Geometry check sheet. Reference: the model listing, model coordinates, mm. Face numbers are marked on the shaded views. A direction names the side the tool comes from. Give positions to 0.01 mm unless a question says otherwise; leave off trailing zeros. Loops run counter-clockwise (first coordinate to the right, second up) from the corner with the lowest first, then second, coordinate; pieces in that order, holes last. Notation, with made-up numbers: (19.25, 70) -> (38.25, 70) arc R33 ccw to (38.25, 103) -> close; hole circle Ø5 at (-20, 60.5). An arc over 180 degrees is marked (long way). One line per item, written item: value. Start each with the question number.
(1) Sectioned sample at D-D, the plane z = 0. Record the cut outline in (x, y).
(2) Draft check along Z on the marked faces 1, 2 and 3. Enter one of: pulls with the +Z half, pulls with the -Z half, needs draft (parallel to the pull), parting line crosses it, or undercut.
(3) Gauge pin test, flat ends, axial feed: pin 1 Ø4 at (x, z) = (-20, -10.5) entering from +Y; pin 2 Ø16.5 at (y, z) = (18, 32.5) entering from -X; pin 3 Ø20.5 at (x, z) = (-11, 43.5) entering from +Y (3 decimals). Record the tip position at first contact, or that the pin passes through.
(4) Sectioned sample at B-B, the plane y = 25.5. Record the cut outline in (x, z) (3 decimals).
(5) Tool access check on the marked faces 4 and 5. Record the directions out of +Z, -Z, +X, -X, +Y, -Y that give a thin tool (end or side, any length) a straight path to the whole face; none if there is none.
(6) Sectioned sample at C-C, the plane x = 0. Record the cut outline in (y, z) (3 decimals).
(7) Sectioned sample at A-A, the plane z = 33.02. Record the cut outline in (x, y) (1 decimal).
(8) Scan lines: line 1 along X through (y, z) = (13.5, 32) (3 decimals); line 2 along Z through (x, y) = (70.5, 17.5); line 3 along Y through (x, z) = (-58.5, -22.5). Record each from-to range of solid material in increasing order. Write a range as from..to.
from build123d import *

# Parameters (mm, degrees)
EXTRUDE_THIN1_DEPTH             = 50.8
FILLET1_RADIUS                  = 4.7625
FILLET1_LENGTH                  = 50.8
FILLET2_R                       = 2.54
CUT_EXTRUDE1_DEPTH              = 97.928543268
CUT_EXTRUDE1_DEPTH_BACK         = 97.928543268
SKETCH5_W                       = 25.4
SKETCH5_H                       = 22.733
CUT_EXTRUDE3_START              = -76.2
SKETCH8_W                       = 50.8
SKETCH8_H                       = 31.75
CUT_EXTRUDE3_DEPTH              = 0.508
M6X1_0_TAPPED_HOLE1_D           = 5
M6X1_0_TAPPED_HOLE1_CSINK_D     = 6.05
M6X1_0_TAPPED_HOLE1_CSINK_ANGLE = 90
MIRROR1_START                   = -50.8
MIRROR1_OUTLINE_W               = 151.384
MIRROR1_OUTLINE_H               = 9.017
MIRROR1_DEPTH                   = 101.6
MIRROR1_2_DEPTH                 = 15.2799999
MIRROR1_START_2                 = 35.5200001
MIRROR1_3_DEPTH                 = 15.2799999
MIRROR1_START_3                 = -30.5199999
MIRROR1_4_DEPTH                 = 5.1199999
MIRROR1_START_4                 = 25.4
MIRROR1_5_DEPTH                 = 5.1199999
MIRROR1_START_5                 = -35.5200001
MIRROR1_6_DEPTH                 = 5.0000002
MIRROR1_START_6                 = 30.5199999
MIRROR1_7_DEPTH                 = 5.0000002
CUT_EXTRUDE2_DEPTH              = 97.529691619
CUT_EXTRUDE2_DEPTH_BACK         = 97.529691619
SKETCH7_R                       = 19.05
M4X0_7_TAPPED_HOLE3_D           = 3.3
M4X0_7_TAPPED_HOLE3_CSINK_D     = 5
M4X0_7_TAPPED_HOLE3_CSINK_ANGLE = 90


with BuildPart() as part:
    # Sketch4 → Extrude-Thin1 (new body)
    with BuildSketch(Plane.XY):
        Polygon((0, 0), (-76.2, 0), (-76.2, 31.75), (-66.675, 31.75), (-66.675, 9.525), (0, 9.525), align=None)
    extrude(amount=EXTRUDE_THIN1_DEPTH)

    # Fillet1: full round fillet: the end face becomes a half cylinder, R = half its width
    fillet1_face = Plane((-71.4375, 31.75, 25.4), x_dir=(0, 0, -1), z_dir=(0, 1, 0))  # on the end face: x along it, z out of the body
    fillet1_slab = fillet1_face.offset(-FILLET1_RADIUS / 2) * Box(FILLET1_LENGTH, 2 * FILLET1_RADIUS, FILLET1_RADIUS, mode=Mode.PRIVATE)  # the body's end, R deep
    fillet1_round = Plane((-71.4375, 26.9875, 25.4), x_dir=(0, 1, 0), z_dir=(0, 0, -1)) * Cylinder(FILLET1_RADIUS, FILLET1_LENGTH, mode=Mode.PRIVATE)  # its axis R under the face
    add(fillet1_slab - fillet1_round, mode=Mode.SUBTRACT)

    # Fillet2
    fillet2_edges = [part.edges().sort_by_distance(p)[0] for p in [
        (-66.675, 9.525, 25.4),
    ]]
    fillet(fillet2_edges, radius=FILLET2_R)

    # Sketch5 → Cut-Extrude1 (cut, two sides: drawn at the far end of the back side and taken through both)
    with BuildSketch(Plane(origin=(0, 0, 0), x_dir=(0, 0, -1), z_dir=(1, 0, 0)).offset(-CUT_EXTRUDE1_DEPTH_BACK)):
        with Locations((-12.7, 20.3835)):
            Rectangle(SKETCH5_W, SKETCH5_H)
    extrude(amount=CUT_EXTRUDE1_DEPTH + CUT_EXTRUDE1_DEPTH_BACK, mode=Mode.SUBTRACT)

    # Sketch8 → Cut-Extrude3 (cut)
    with BuildSketch(Plane(origin=(0, 0, 0), x_dir=(0, 0, -1), z_dir=(1, 0, 0)).offset(CUT_EXTRUDE3_START)):
        with Locations((-25.4, 15.875)):
            Rectangle(SKETCH8_W, SKETCH8_H)
    extrude(amount=CUT_EXTRUDE3_DEPTH, mode=Mode.SUBTRACT)

    # M6x1.0 Tapped Hole1 (through all)
    with Locations(Plane.ZY.offset(75.692)):
        with Locations((33.02, 17.145)):
            CounterSinkHole(M6X1_0_TAPPED_HOLE1_D / 2, M6X1_0_TAPPED_HOLE1_CSINK_D / 2, counter_sink_angle=M6X1_0_TAPPED_HOLE1_CSINK_ANGLE)

    # Mirror1: read off the stored shape, not the designer's step
    # Mirror1 outline → Mirror1 (add)
    with BuildSketch(Plane.XY.offset(MIRROR1_START)):
        with Locations((0, 4.5085)):
            Rectangle(MIRROR1_OUTLINE_W, MIRROR1_OUTLINE_H)
    extrude(amount=MIRROR1_DEPTH)

    # Mirror1 2 outline → Mirror1 2 (add)
    with BuildSketch(Plane.XY.offset(MIRROR1_START)):
        with BuildLine():
            Line((-66.675, 12.065), (-66.675, 26.9875))
            ThreePointArc((-66.675, 26.9875), (-70.337647737, 31.621259947), (-75.692, 29.127742042))
            Line((-75.692, 29.127742042), (-75.692, 9.017))
            Line((-75.692, 9.017), (75.692, 9.017))
            Line((75.692, 9.017), (75.692, 29.127742042))
            ThreePointArc((75.692, 29.127742042), (70.337647737, 31.621259947), (66.675, 26.9875))
            Line((66.675, 26.9875), (66.675, 12.065))
            ThreePointArc((66.675, 12.065), (65.931051224, 10.268948776), (64.135, 9.525))
            Line((64.135, 9.525), (-64.135, 9.525))
            ThreePointArc((-64.135, 9.525), (-65.931051224, 10.268948776), (-66.675, 12.065))
        make_face()
    extrude(amount=MIRROR1_2_DEPTH)

    # Mirror1 3 outline → Mirror1 3 (add)
    with BuildSketch(Plane.XY.offset(MIRROR1_START_2)):
        with BuildLine():
            Line((0, 9.525), (0, 9.017))
            Line((0, 9.017), (75.692, 9.017))
            Line((75.692, 9.017), (75.692, 29.127742042))
            ThreePointArc((75.692, 29.127742042), (70.337647737, 31.621259947), (66.675, 26.9875))
            Line((66.675, 26.9875), (66.675, 12.065))
            ThreePointArc((66.675, 12.065), (65.931051224, 10.268948776), (64.135, 9.525))
            Line((64.135, 9.525), (0, 9.525))
        make_face()
    extrude(amount=MIRROR1_3_DEPTH)

    # Mirror1 4 outline → Mirror1 4 (add)
    with BuildSketch(Plane.XY.offset(MIRROR1_START_3)):
        with BuildLine():
            Line((-66.675, 12.065), (-66.675, 26.9875))
            ThreePointArc((-66.675, 26.9875), (-70.337647737, 31.621259947), (-75.692, 29.127742042))
            Line((-75.692, 29.127742042), (-75.692, 9.017))
            Line((-75.692, 9.017), (75.692, 9.017))
            Line((75.692, 9.017), (75.692, 29.127742042))
            ThreePointArc((75.692, 29.127742042), (70.337647737, 31.621259947), (66.675, 26.9875))
            Line((66.675, 26.9875), (66.675, 12.065))
            ThreePointArc((66.675, 12.065), (65.931051224, 10.268948776), (64.135, 9.525))
            Line((64.135, 9.525), (-64.135, 9.525))
            ThreePointArc((-64.135, 9.525), (-65.931051224, 10.268948776), (-66.675, 12.065))
        make_face()
    extrude(amount=MIRROR1_4_DEPTH)

    # Mirror1 5 outline → Mirror1 5 (add)
    with BuildSketch(Plane.XY.offset(MIRROR1_START_4)):
        with BuildLine():
            Line((0, 9.525), (0, 9.017))
            Line((0, 9.017), (75.692, 9.017))
            Line((75.692, 9.017), (75.692, 29.127742042))
            ThreePointArc((75.692, 29.127742042), (70.337647737, 31.621259947), (66.675, 26.9875))
            Line((66.675, 26.9875), (66.675, 12.065))
            ThreePointArc((66.675, 12.065), (65.931051224, 10.268948776), (64.135, 9.525))
            Line((64.135, 9.525), (0, 9.525))
        make_face()
    extrude(amount=MIRROR1_5_DEPTH)

    # Mirror1 6 outline → Mirror1 6 (add)
    with BuildSketch(Plane.XY.offset(MIRROR1_START_5)):
        with BuildLine():
            Line((-66.675, 12.065), (-66.675, 26.9875))
            ThreePointArc((-66.675, 26.9875), (-70.337647737, 31.621259947), (-75.692, 29.127742042))
            Line((-75.692, 29.127742042), (-75.692, 9.017))
            Line((-75.692, 9.017), (75.692, 9.017))
            Line((75.692, 9.017), (75.692, 29.127742042))
            ThreePointArc((75.692, 29.127742042), (70.337647737, 31.621259947), (66.675, 26.9875))
            Line((66.675, 26.9875), (66.675, 12.065))
            ThreePointArc((66.675, 12.065), (65.931051224, 10.268948776), (64.135, 9.525))
            Line((64.135, 9.525), (-64.135, 9.525))
            ThreePointArc((-64.135, 9.525), (-65.931051224, 10.268948776), (-66.675, 12.065))
        make_face()
    extrude(amount=MIRROR1_6_DEPTH)

    # Mirror1 7 outline → Mirror1 7 (add)
    with BuildSketch(Plane.XY.offset(MIRROR1_START_6)):
        with BuildLine():
            Line((0, 9.525), (0, 9.017))
            Line((0, 9.017), (75.692, 9.017))
            Line((75.692, 9.017), (75.692, 29.127742042))
            ThreePointArc((75.692, 29.127742042), (70.337647737, 31.621259947), (66.675, 26.9875))
            Line((66.675, 26.9875), (66.675, 12.065))
            ThreePointArc((66.675, 12.065), (65.931051224, 10.268948776), (64.135, 9.525))
            Line((64.135, 9.525), (0, 9.525))
        make_face()
    extrude(amount=MIRROR1_7_DEPTH)

    # Mirror1 8 outline → Mirror1 8 (revolve, cut)
    with BuildSketch(Plane(origin=(0, 17.145, 33.02), x_dir=(0, 1, 0), z_dir=(0, 0, -1))):
        Polygon((0, 66.675), (2.5, 66.675), (2.5, 75.167), (3.025, 75.692), (0, 75.692), align=None)
    revolve(axis=Axis((0, 17.145, 33.02), (1, 0, 0)), mode=Mode.SUBTRACT)

    # Mirror1 9 outline → Mirror1 9 (revolve, cut)
    with BuildSketch(Plane(origin=(0, 17.145, -33.02), x_dir=(0, 1, 0), z_dir=(0, 0, -1))):
        Polygon((2.5, -75.167), (2.5, -66.675), (0, -66.675), (0, -75.692), (3.025, -75.692), align=None)
        Polygon((0, 66.675), (2.5, 66.675), (2.5, 75.167), (3.025, 75.692), (0, 75.692), align=None)
    revolve(axis=Axis((0, 17.145, -33.02), (1, 0, 0)), mode=Mode.SUBTRACT)

    # Sketch7 → Cut-Extrude2 (cut, two sides: drawn at the far end of the back side and taken through both)
    with BuildSketch(Plane(origin=(0, 0, 0), x_dir=(1, 0, 0), z_dir=(0, 1, 0)).offset(-CUT_EXTRUDE2_DEPTH_BACK)):
        with Locations(Location((0, 0, 0), (0, 0, 270))):
            Circle(SKETCH7_R)
    extrude(amount=CUT_EXTRUDE2_DEPTH + CUT_EXTRUDE2_DEPTH_BACK, mode=Mode.SUBTRACT)

    # M4x0.7 Tapped Hole3 (through all)
    with Locations(Plane(origin=(0, 9.017, 0), x_dir=(1, 0, 0), z_dir=(0, 1, 0))):
        with Locations((38.608, -12.446), (-38.608, -12.446), (-38.608, 12.446), (38.608, 12.446)):
            CounterSinkHole(M4X0_7_TAPPED_HOLE3_D / 2, M4X0_7_TAPPED_HOLE3_CSINK_D / 2, counter_sink_angle=M4X0_7_TAPPED_HOLE3_CSINK_ANGLE)


solid = part.part
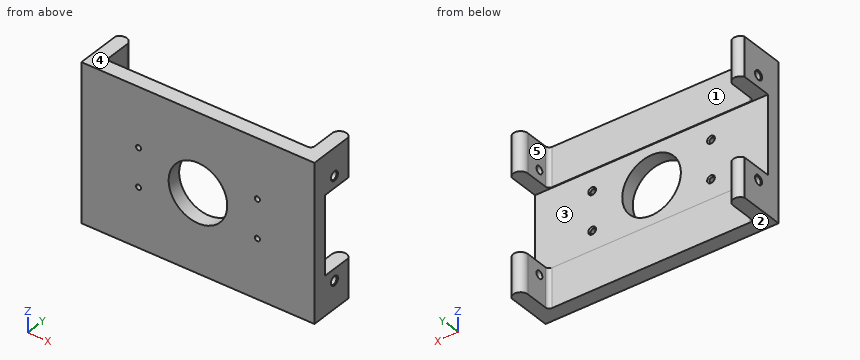
Calculated:
1. outline: (-75.69, 0) -> (-19.05, 0) -> (-19.05, 9.02) -> (-75.69, 9.02) -> close; (19.05, 0) -> (75.69, 0) -> (75.69, 9.02) -> (19.05, 9.02) -> close
2. face 1: needs draft
2. face 2: pulls with the -Z half
2. face 3: undercut
3. pin 1: stops at y = 9.02
3. pin 2: stops at x = -75.69
3. pin 3: stops at y = 9.525
4. outline: (-75.692, -50.8) -> (-66.675, -50.8) -> (-66.675, -25.4) -> (-75.692, -25.4) -> close; (-75.692, 25.4) -> (-66.675, 25.4) -> (-66.675, 50.8) -> (-75.692, 50.8) -> close; (66.675, -50.8) -> (75.692, -50.8) -> (75.692, -25.4) -> (66.675, -25.4) -> close; (66.675, 25.4) -> (75.692, 25.4) -> (75.692, 50.8) -> (66.675, 50.8) -> close
5. face 4: +Z, +X, -X, +Y, -Y
5. face 5: +Z, -Z, +Y
6. outline: (0, -50.8) -> (9.525, -50.8) -> (9.525, -25.4) -> (9.017, -25.4) -> (9.017, -19.05) -> (0, -19.05) -> close; (0, 19.05) -> (9.017, 19.05) -> (9.017, 25.4) -> (9.525, 25.4) -> (9.525, 50.8) -> (0, 50.8) -> close
7. outline: (-75.7, 0) -> (75.7, 0) -> (75.7, 14.1) -> (75.2, 14.6) -> (66.7, 14.6) -> (66.7, 12.1) arc R2.5 cw to (64.1, 9.5) -> (-64.1, 9.5) arc R2.5 cw to (-66.7, 12.1) -> (-66.7, 14.6) -> (-75.2, 14.6) -> (-75.7, 14.1) -> close; (-75.7, 20.2) -> (-75.2, 19.6) -> (-66.7, 19.6) -> (-66.7, 27) arc R4.8 ccw to (-75.7, 29.1) -> close; (66.7, 19.6) -> (75.2, 19.6) -> (75.7, 20.2) -> (75.7, 29.1) arc R4.8 ccw to (66.7, 27) -> close
8. line 1: x = -75.692..-66.675, 66.675..75.692
8. line 2: z = -50.8..-35.49, -30.55..-25.4, 25.4..30.55, 35.49..50.8
8. line 3: y = 0..9.02
